CAD build for the part. Positions are in the model's coordinates, mm. Face numbers are marked on the shaded views. A direction names the side the tool comes from. Give positions to 0.01 mm unless a question says otherwise; leave off trailing zeros. Order: outer loops, then holes, each group sorted by start corner. A loop starts at its lowest first (then second) coordinate and runs counter-clockwise, first axis right, second up. Notation, with made-up numbers: M 69,68.5 L 108,68.5 A5 cw 108,75.5 Z; hole C -19,72 d10. An arc over 180 degrees is marked long. Put each result on its own line as item: value. Start each with the question number.
1) Cut at A-A (x = -52.5). Write the cut outline in (y, z).
2) Cut at D-D (x = 2). Write the cut outline in (y, z).
3) Tool access for the marked faces 1 and 2: list every direction of +Z, -Z, +X, -X, +Y, -Y with a clear straight run to the whole face (end or side of a thin tool).
4) Drill centre lines: line 1 (X direction, y = 1.15, z = -52.5); line 2 (X direction, y = 0.85, z = -1.5); line 3 (Z direction, x = -45.5, y = 1.25). Where is each one in solid material? Low to high. Write a range as [from, to].
5) Cut at C-C (z = -14.5). Write the cut outline in (x, y).
6) Pin check, flat tips, straight feed: pin 1 (0.5 mm diameter, centred on y = 2.5, z = 49, fed in from -X); pin 2 (3 mm diameter, centred on x = -43.13, z = -35.63, fed in from -Y); pin 3 (0.5 mm diameter, centred on x = -52.5, y = 2.5, fed in from +Z); pin 4 (1.1 mm diameter, centred on x = 16, y = 2.5, fed in from +Z). Stop position of each tip, or through.
7) Cut at B-B (z = 52.5). Write the cut outline in (x, y), and give its area (3 significant figures).
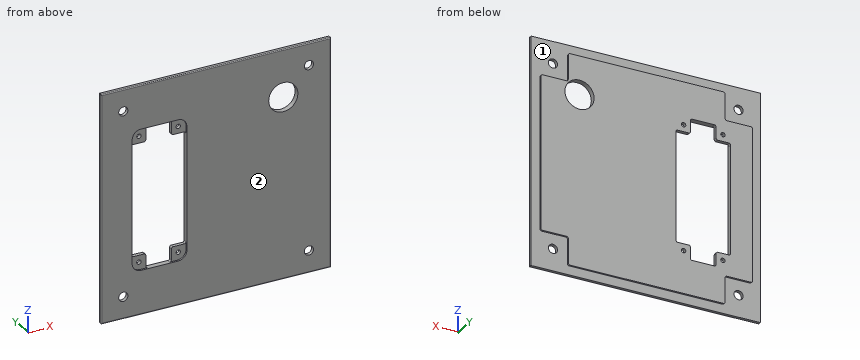
```python
from build123d import *

# Parameters (mm, degrees)
SKETCH_1_W          = 130
SKETCH_1_H          = 130
EXTRUDE_1_DEPTH     = 3
SKETCH_2_R          = 2.6
CUT_EXTRUDE_1_DEPTH = 92.972822073
SKETCH_4_W          = 20.650518397
SKETCH_4_H          = 20.951555191
CUT_EXTRUDE_2_DEPTH = 1
SKETCH_5_W          = 88.698963206
SKETCH_5_H          = 5.1
SKETCH_5_W_2        = 5.1
SKETCH_5_H_2        = 88.096889618
CUT_EXTRUDE_3_DEPTH = 1
CUT_EXTRUDE_4_DEPTH = 3
EXTRUDE_START       = -2
SKETCH_7_R          = 1.25
EXTRUDE_2_DEPTH     = 2
FILLET_1_R          = 1
SKETCH_15_R         = 8.25
CUT_EXTRUDE_9_DEPTH = 92.972822073
CHAMFER_2_SIZE      = 0.2
FILLET_2_R          = 0.5
FILLET_3_R          = 1
FILLET_4_R          = 1


with BuildPart() as part:
    # 草图1 → 凸台-拉伸1 (new body)
    with BuildSketch(Plane(origin=(0, 0, 0), x_dir=(1, 0, 0), z_dir=(0, 1, 0))):
        Rectangle(SKETCH_1_W, SKETCH_1_H)
    extrude(amount=EXTRUDE_1_DEPTH)

    # 草图2 → 切除-拉伸1 (cut, through all)
    with BuildSketch(Plane(origin=(0, 3, 0), x_dir=(1, 0, 0), z_dir=(0, 1, 0))):
        with Locations(Location((52.5, 52.5, 0), (0, 0, 270))):
            Circle(SKETCH_2_R)
        with Locations(Location((52.5, -52.5, 0), (0, 0, 270))):
            Circle(SKETCH_2_R)
        with Locations(Location((-52.5, -52.5, 0), (0, 0, 270))):
            Circle(SKETCH_2_R)
        with Locations(Location((-52.5, 52.5, 0), (0, 0, 270))):
            Circle(SKETCH_2_R)
    extrude(amount=-CUT_EXTRUDE_1_DEPTH, mode=Mode.SUBTRACT)

    # 草图4 → 切除-拉伸2 (cut)
    with BuildSketch(Plane(origin=(0, 3, 0), x_dir=(1, 0, 0), z_dir=(0, 1, 0))):
        with Locations((54.674740802, 54.524222405)):
            Rectangle(SKETCH_4_W, SKETCH_4_H)
        with Locations((-54.674740802, -54.524222405)):
            Rectangle(SKETCH_4_W, SKETCH_4_H)
        with Locations((54.674740802, -54.524222405)):
            Rectangle(SKETCH_4_W, SKETCH_4_H)
        with Locations((-54.674740802, 54.524222405)):
            Rectangle(SKETCH_4_W, SKETCH_4_H)
    extrude(amount=-CUT_EXTRUDE_2_DEPTH, mode=Mode.SUBTRACT)

    # 草图5 → 切除-拉伸3 (cut)
    with BuildSketch(Plane(origin=(0, 3, 0), x_dir=(1, 0, 0), z_dir=(0, 1, 0))):
        with Locations((0, 62.45)):
            Rectangle(SKETCH_5_W, SKETCH_5_H)
        with Locations((62.45, 0)):
            Rectangle(SKETCH_5_W_2, SKETCH_5_H_2)
        with Locations((0, -62.45)):
            Rectangle(SKETCH_5_W, SKETCH_5_H)
        with Locations((-62.45, 0)):
            Rectangle(SKETCH_5_W_2, SKETCH_5_H_2)
    extrude(amount=-CUT_EXTRUDE_3_DEPTH, mode=Mode.SUBTRACT)

    # 草图6 → 切除-拉伸4 (cut)
    with BuildSketch(Plane(origin=(0, 0, 0), x_dir=(-1, 0, 0), z_dir=(0, -1, 0))):
        with BuildLine():
            Line((47.5, -35), (47.5, 35))
            ThreePointArc((47.5, 35), (46.035533906, 38.535533906), (42.5, 40))
            Line((42.5, 40), (21.5, 40))
            ThreePointArc((21.5, 40), (17.964466094, 38.535533906), (16.5, 35))
            Line((16.5, 35), (16.5, -35))
            ThreePointArc((16.5, -35), (17.964466094, -38.535533906), (21.5, -40))
            Line((21.5, -40), (42.5, -40))
            ThreePointArc((42.5, -40), (46.035533906, -38.535533906), (47.5, -35))
        make_face()
    extrude(amount=-CUT_EXTRUDE_4_DEPTH, mode=Mode.SUBTRACT)

    # 草图7 → 凸台-拉伸2 (add)
    # profile 1 of 4: a face of its own
    with BuildSketch(Plane(origin=(0, 3, 0), x_dir=(1, 0, 0), z_dir=(0, 1, 0)).offset(EXTRUDE_START)):
        with BuildLine():
            Line((-24.75, 40), (-24.75, 31.75))
            Line((-24.75, 31.75), (-16.5, 31.75))
            Line((-16.5, 31.75), (-16.5, 35))
            ThreePointArc((-16.5, 35), (-17.964466094, 38.535533906), (-21.5, 40))
            Line((-21.5, 40), (-24.75, 40))
        make_face()
        with Locations(Location((-20.872307757, 35.627692243, 0), (0, 0, 270))):
            Circle(SKETCH_7_R, mode=Mode.SUBTRACT)
    # profile 2 of 4: a face of its own
    with BuildSketch(Plane(origin=(0, 3, 0), x_dir=(1, 0, 0), z_dir=(0, 1, 0)).offset(EXTRUDE_START)):
        with BuildLine():
            Line((-16.5, -31.75), (-24.75, -31.75))
            Line((-24.75, -31.75), (-24.75, -40))
            Line((-24.75, -40), (-21.5, -40))
            ThreePointArc((-21.5, -40), (-17.964466094, -38.535533906), (-16.5, -35))
            Line((-16.5, -35), (-16.5, -31.75))
        make_face()
        with Locations(Location((-20.872307757, -35.627692243, 0), (0, 0, 270))):
            Circle(SKETCH_7_R, mode=Mode.SUBTRACT)
    # profile 3 of 4: a face of its own
    with BuildSketch(Plane(origin=(0, 3, 0), x_dir=(1, 0, 0), z_dir=(0, 1, 0)).offset(EXTRUDE_START)):
        with BuildLine():
            Line((-39.25, -40), (-39.25, -31.75))
            Line((-39.25, -31.75), (-47.5, -31.75))
            Line((-47.5, -31.75), (-47.5, -35))
            ThreePointArc((-47.5, -35), (-46.035533906, -38.535533906), (-42.5, -40))
            Line((-42.5, -40), (-39.25, -40))
        make_face()
        with Locations(Location((-43.127692243, -35.627692243, 0), (0, 0, 270))):
            Circle(SKETCH_7_R, mode=Mode.SUBTRACT)
    # profile 4 of 4: a face of its own
    with BuildSketch(Plane(origin=(0, 3, 0), x_dir=(1, 0, 0), z_dir=(0, 1, 0)).offset(EXTRUDE_START)):
        with BuildLine():
            Line((-47.5, 31.75), (-39.25, 31.75))
            Line((-39.25, 31.75), (-39.25, 40))
            Line((-39.25, 40), (-42.5, 40))
            ThreePointArc((-42.5, 40), (-46.035533906, 38.535533906), (-47.5, 35))
            Line((-47.5, 35), (-47.5, 31.75))
        make_face()
        with Locations(Location((-43.127692243, 35.627692243, 0), (0, 0, 270))):
            Circle(SKETCH_7_R, mode=Mode.SUBTRACT)
    extrude(amount=EXTRUDE_2_DEPTH)

    # 圆角1
    fillet_1_edges = [part.edges().sort_by_distance(p)[0] for p in [
        (-24.75, 2, -31.75),
        (-39.25, 2, -31.75),
        (-39.25, 2, 31.75),
        (-24.75, 2, 31.75),
    ]]
    fillet(fillet_1_edges, radius=FILLET_1_R)

    # 草图15 → 切除-拉伸9 (cut, through all)
    with BuildSketch(Plane(origin=(0, 0, 0), x_dir=(-1, 0, 0), z_dir=(0, -1, 0))):
        with Locations(Location((-38, -38, 0), (0, 0, 90))):
            Circle(SKETCH_15_R)
    extrude(amount=-CUT_EXTRUDE_9_DEPTH, mode=Mode.SUBTRACT)

    # 倒角2
    chamfer_2_edges = [part.edges().sort_by_distance(p)[0] for p in [
        (65, 1, 65),
        (-65, 1, 65),
        (-65, 1, -65),
        (65, 1, -65),
    ]]
    chamfer(chamfer_2_edges, length=CHAMFER_2_SIZE)

    # 圆角2
    # the kernel refuses this fillet: 0.5 mm, written as the material it takes off along each edge
    with BuildSketch(Plane(origin=(-66.05, 0, -65), x_dir=(0, 0, 1), z_dir=(1, 0, 0)), Plane(origin=(-65, 0, 66.05), x_dir=(1, 0, 0), z_dir=(0, 0, -1)), Plane(origin=(66.05, 0, 65), x_dir=(0, 0, -1), z_dir=(-1, 0, 0)), Plane(origin=(65, 0, -66.05), x_dir=(-1, 0, 0), z_dir=(0, 0, 1))) as fillet_2_piece_1:
        with BuildLine():
            CenterArc((FILLET_2_R, -FILLET_2_R), FILLET_2_R, 90, 90)
            Line((0, -FILLET_2_R), (0, 0))
            Line((0, 0), (FILLET_2_R, 0))
        make_face()
    extrude(amount=132.1, mode=Mode.SUBTRACT)

    # 圆角3
    fillet_3_edges = [part.edges().sort_by_distance(p)[0] for p in [
        (59.9, 2.5, 44.048444809),
        (59.9, 2.5, -44.048444809),
        (-44.349481603, 2.5, -59.9),
        (44.349481603, 2.5, -59.9),
        (44.349481603, 2.5, 59.9),
        (-44.349481603, 2.5, 59.9),
        (-59.9, 2.5, 44.048444809),
        (-59.9, 2.5, -44.048444809),
        (-44.349481603, 2.5, -44.048444809),
        (-44.349481603, 2.5, 44.048444809),
        (44.349481603, 2.5, 44.048444809),
        (44.349481603, 2.5, -44.048444809),
    ]]
    fillet(fillet_3_edges, radius=FILLET_3_R)

    # 圆角4
    fillet_4_edges = [part.edges().sort_by_distance(p)[0] for p in [
        (-24.75, 2, -40),
        (-16.5, 2, -31.75),
        (-47.5, 2, -31.75),
        (-39.25, 2, -40),
        (-39.25, 2, 40),
        (-47.5, 2, 31.75),
        (-16.5, 2, 31.75),
        (-24.75, 2, 40),
    ]]
    fillet(fillet_4_edges, radius=FILLET_4_R)


solid = part.part
```
Solution:
1. outline: M 0,-64.5 A0.5 ccw 0.5,-65 L 2,-65 L 2,-55.1 L 0,-55.1 Z; M 0,-49.9 L 2,-49.9 L 2,-44.05 L 3,-44.05 L 3,44.05 L 2,44.05 L 2,49.9 L 0,49.9 Z; M 0,55.1 L 2,55.1 L 2,65 L 0.5,65 A0.5 ccw 0,64.5 Z
2. outline: M 0,-64.5 A0.5 ccw 0.5,-65 L 2,-65 L 2,-59.9 L 3,-59.9 L 3,59.9 L 2,59.9 L 2,65 L 0.5,65 A0.5 ccw 0,64.5 Z
3. face 1: +Y
3. face 2: +Z, -Z, +X, -X, -Y
4. line 1: [-65, -55.1], [-49.9, 49.9], [55.1, 65]
4. line 2: [-65, -47.5], [-16.5, 65]
4. line 3: [-65, -31.75], [31.75, 65]
5. outline: M -65,0.5 A0.5 ccw -64.5,0 L -47.5,0 L -47.5,3 L -59.9,3 L -59.9,2 L -65,2 Z; M -16.5,0 L 64.5,0 A0.5 ccw 65,0.5 L 65,2 L 59.9,2 L 59.9,3 L -16.5,3 Z
6. pin 1: x = -44.35
6. pin 2: y = 1
6. pin 3: z = 44.05
6. pin 4: z = 65
7. outline: M -65,0.5 A0.5 ccw -64.5,0 L -55.1,0 L -55.1,2 L -65,2 Z; M -49.9,0 L 49.9,0 L 49.9,2 L 44.35,2 L 44.35,3 L -44.35,3 L -44.35,2 L -49.9,2 Z; M 55.1,0 L 64.5,0 A0.5 ccw 65,0.5 L 65,2 L 55.1,2 Z
7. area: 328 mm²
